Autodesk Inventor part; units mm, degrees
ref_plane "YZ Plane" through (0, 0, 0) normal (1, 0, 0) x (0, 1, 0)
ref_plane "XZ Plane" through (0, 0, 0) normal (0, 1, 0) x (-1, 0, 0)
sketch "Sketch1" plane through (0, 0, 0) normal (0, 0, 1) x (1, 0, 0)
  circle A0 centre (0, 0) radius 2.5
  circle A1 centre (0, 0) radius 4
  line L0 (-3.5063, 3.5) -> (5.715, 3.5) construction
  line L1 (-3.4532, 4.1) -> (5.7681, 4.1) construction
  dimension "d0" = 5
  dimension "d1" = 0.6
  dimension "d2" = 0.1
  dimension "d3" = 1
extrude "Extrusion1" add sketch "Sketch1" along normal blind 10
sketch "Sketch2" plane through (0, 0, 0) normal (1, 0, 0) x (0, 1, 0)
  line L0 (4, 10) -> (-4, 10)
  line L1 (-4, 0) -> (4, 0)
  line L2 (4, 10) -> (4, 8.7612)
  line L3 (4, 0) -> (4, 10)
  circle A0 centre (3.8, 8.2731) radius 0.3
  line L4 (4, 8.7612) -> (3.25, 8.2731)
  line L5 (3.25, 8.2731) -> (4, 7.785)
  line L6 (2.5, 0) -> (2.5, 10)
  line L7 (0, -2) -> (0, 12)
  point P0 (0, 0)
  dimension "d6" = 0.6
  dimension "d7" = 0.1
  dimension "d8" = 0.75
revolve "Revolution1" cut sketch "Sketch2" angle 360 about axis through (0, 0, -10) along (0, 0, 1) picked at (3.9033, 8.3516) contours L3 A0 L4 | L3 A0 | A0 L5 L4 | L3 L5 A0
ref_plane "Work Plane1" through (0, 3.25, 8.2731) normal (0, 0, 1) x (1, 0, 0)
sketch "Sketch4" plane through (0, 3.25, 8.2731) normal (0, 0, 1) x (1, 0, 0)
  line L0 (-1.6699, 0.85) -> (1.5938, 0.85) construction
  line L1 (-1.4284, 0.3) -> (1.8353, 0.3) construction
  circle A0 centre (0, -3.25) radius 4
  circle A1 centre (0, -3.25) radius 3.25
  line L2 (0, -3.25) -> (-0.2833, -0.0124)
  line L3 (0, -3.25) -> (0.2833, -0.0124)
  arc A2 (0.2833, -0.0124) -> (-0.2833, -0.0124) centre (0, -3.25) ccw
  line L4 (-0.2833, -0.0124) -> (0, 0.3)
  line L5 (0, 0.3) -> (0.2833, -0.0124)
  point P0 (0, 0)
  dimension "d16" = 0.55
  dimension "d17" = 0.1
  dimension "d18" = 10
extrude "Extrusion3" add sketch "Sketch4" along normal through all both and the other way through all contours A1 L4 L5
sketch "Sketch3" plane through (0, 3.25, 8.2731) normal (0, 0, 1) x (1, 0, 0)
  line L0 (0, -3.25) -> (-0.1745, 0.7462) construction
  circle A0 centre (0, -3.25) radius 4
  line L1 (0, -3.25) -> (0.1745, 0.7462) construction
  arc A1 (0.1745, 0.7462) -> (-0.1745, 0.7462) centre (0, -3.25) ccw
  circle A2 centre (0, -3.25) radius 3.25
  arc A3 (0.1418, -0.0031) -> (-0.1418, -0.0031) centre (0, -3.25) ccw
  line L2 (-0.1745, 0.7462) -> (-0.1418, -0.0031)
  line L3 (0.1418, -0.0031) -> (0.1745, 0.7462)
  line L4 (0, 0.75) -> (-0.1418, -0.0031)
  line L5 (0, 0.75) -> (0.1418, -0.0031)
  point P0 (0, 0)
  dimension "d10" = 5
pattern_circular "Circular Pattern2" count 24 over 360 about axis through (0, 0, -10) along (0, 0, 1) of "Extrusion3"
properties part number "Thoughts for a new driver gear"
Design review of the part built by this model. Coordinates are the model's own, in mm. Coordinates: 2 decimals unless noted, no trailing zeros. Write each loop counter-clockwise with the first axis right and the second up, starting at its lowest first coordinate (ties: lowest second). Pieces come first, ordered by that corner, then holes. Notation, with made-up numbers: (68.25, 40.5) - (77.25, 40.5) arc R33 ccw to (77.25, 74.5) - close; hole circle Ø10 at (38, 71). An arc over 180 degrees is marked (long way). One line per item, written item: value.
1) Add section A-A (z = 4.75). State the section outline as (x, y) points.
Answer sheet:
outline: circle Ø8 at (0, 0); hole circle Ø5 at (0, 0)
2) To check wall thickness, follow probe 1 along Y at (x, z) = (0, 6.5); probe 2 along Z at (x, y) = (-2.25, -2.75); probe 3 along X at (y, z) = (0.5, 1). State the ranges of each line that lie inside material, in increasing order.
Answer sheet:
probe 1: y = -4 to -2.5, 2.5 to 4
probe 2: z = 0 to 8.08, 8.47 to 10
probe 3: x = -3.97 to -2.45, 2.45 to 3.97
3) Insertion check: pin 1 (2 mm diameter, centred on y = -2.5, z = 4, fed in from -X); pin 2 (1.5 mm diameter, centred on x = -1.5, z = 4, fed in from +Y); pin 3 (2 mm diameter, centred on x = 2.5, z = 5.5, fed in from -Y). Each pin has a flat end and moves straight along its axis. Give the tip position at first contact, or say it passes through.
Answer sheet:
pin 1: stops at x = -3.71
pin 2: stops at y = 3.93
pin 3: stops at y = -3.71
